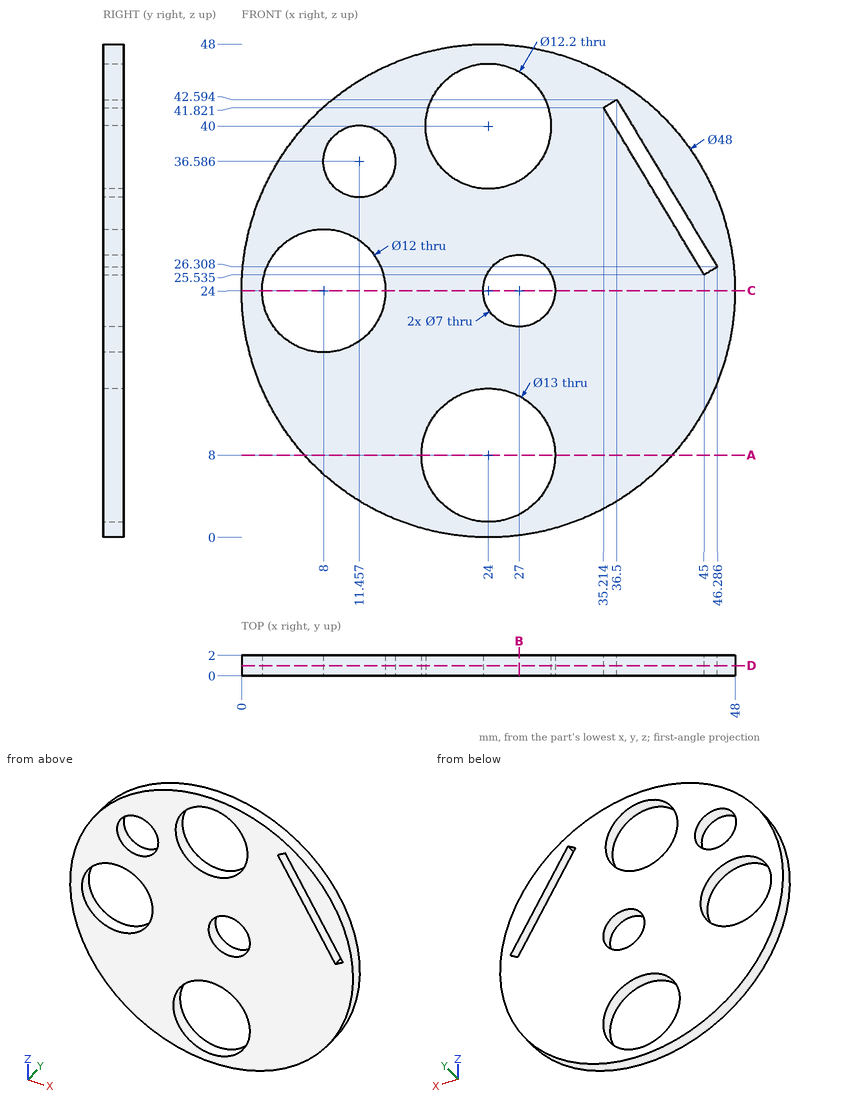
The figure shows three views and two pictorial views of one solid part (mm, origin at its lowest corner). Answer the questions. Coordinates: 2 decimals unless noted, no trailing zeros. Write each loop counter-clockwise with the first axis right and the second up, starting at its lowest first coordinate (ties: lowest second). Pieces come first, ordered by that corner, then holes. Notation, with made-up numbers: (69.5, 46.25) -> (88.5, 46.25) arc R22 cw to (88.5, 67.25) -> close; hole circle Ø1 at (-14, 85.5). An arc over 180 degrees is marked (long way). Return JSON: item names as keys, results as strings.
(1) The part is cut by section C-C on z = 24. Give the vertices of the cut face in (x, y).
Answers below:
{"outline": "(0, 0) -> (2, 0) -> (2, 2) -> (0, 2) -> close; (14, 0) -> (23.5, 0) -> (23.5, 2) -> (14, 2) -> close; (30.5, 0) -> (48, 0) -> (48, 2) -> (30.5, 2) -> close"}
(2) The part is cut by section B-B on x = 27. Give the vertices of the cut face in (y, z).
Answers below:
{"outline": "(0, 0.19) -> (2, 0.19) -> (2, 2.23) -> (0, 2.23) -> close; (0, 13.77) -> (2, 13.77) -> (2, 20.5) -> (0, 20.5) -> close; (0, 27.5) -> (2, 27.5) -> (2, 34.69) -> (0, 34.69) -> close; (0, 45.31) -> (2, 45.31) -> (2, 47.81) -> (0, 47.81) -> close"}
(3) Each of these flat-tipped pins is pushed along its axis until it touches: P1, Ø11.5, axis at x = 24, z = 8, coming from the +Y side (3 decimals); P2, Ø1, axis at y = 0.5, z = 28, coming from the +X side. Where does it stop, or does it pass through?
Answers below:
{"P1": "through", "P2": "x = 47.74"}
(4) Consider line 1 along X through (y, z) = (1.2, 24); line 2 along Z through (x, y) = (9, 0.8) (1 decimal); line 3 along Z through (x, y) = (22.5, 0.9) (1 decimal). Determine where each line is inside the solid, lowest interval first. Write a range as from..to.
Answers below:
{"line 1": "0..2, 14..23.5, 30.5..48", "line 2": "5.3..18.1, 29.9..34.1, 39.1..42.7", "line 3": "0..1.7, 14.3..34.1, 45.9..48"}
(5) The part is cut by section D-D on y = 1. Give the vertices of the cut face in (x, z) (1 decimal), then the cut area to 3 significant figures.
Answers below:
{"outline": "circle Ø48 at (24, 24); hole circle Ø12 at (8, 24); hole circle Ø7 at (11.5, 36.6); hole circle Ø13 at (24, 8); hole circle Ø12.2 at (24, 40); hole circle Ø7 at (27, 24); hole (35.2, 41.8) -> (45, 25.5) -> (46.3, 26.3) -> (36.5, 42.6) -> close", "area": "1,340 mm^2"}
(6) The part is cut by section A-A on z = 8. Give the vertices of the cut face in (x, y).
Answers below:
{"outline": "(6.11, 0) -> (17.5, 0) -> (17.5, 2) -> (6.11, 2) -> close; (30.5, 0) -> (41.89, 0) -> (41.89, 2) -> (30.5, 2) -> close"}
